Work out the finished part from the listing and answer in its coordinate system (mm). Coordinates: 2 decimals unless noted, no trailing zeros. Order: outer loops, then holes, each group sorted by start corner. A loop starts at its lowest first (then second) coordinate and runs counter-clockwise, first axis right, second up. Notation, with made-up numbers: (62.5, 55.5) - (102.5, 55.5) arc R18 ccw to (102.5, 59.5) - close; hole circle Ø5 at (88.25, 83). An arc over 180 degrees is marked (long way). Answer as a JSON object with one key per item and string values. Group by question number.
1) Section A-A (y = -0.95) is taken. Give the vertices of the cut face in (x, z) (1 decimal).
2) Find the intervals of material crossed by line 1 along X through (y, z) = (-0.1, 0); line 2 along X through (y, z) = (0.5, 0.75); line 3 along Z through (x, y) = (3.5, 0.9), in increasing order.
3) The mould has two halves that part along X. Classify faces 1 (the face through (-0.966, 0.015, -1.26)), 2 (the face through (3.563, -1.363, 2.046)), 3 (the face through (-3.962, 0, 0)), 4 (the face through (0.01, 1.363, 4.109)): released by +X, released by -X, zero draft, split by the parting line, or undercut.
4) This flat-tipped pin is pushed along its axis until it touches: P1, Ø3, axis at x = 0, z = 0, coming from the +Y side. Where does it stop, or does it pass through?
from build123d import *

# Parameters (mm, degrees)
BOSS_EXTRUDE1_DEPTH = 1.4478
SKETCH2_R           = 1.5875
CUT_EXTRUDE1_DEPTH  = 7.709639692
CHAMFER2_SIZE       = 0.381


with BuildPart() as part:
    # Sketch1 → Boss-Extrude1 (new, symmetric)
    with BuildSketch(Plane(origin=(0, 0, 0), x_dir=(1, 0, 0), z_dir=(0, 1, 0))):
        Polygon((0, -4.575385413), (3.9624, -2.287692707), (3.9624, 2.287692707), (0, 4.575385413), (-3.9624, 2.287692707), (-3.9624, -2.287692707), align=None)
    extrude(amount=BOSS_EXTRUDE1_DEPTH, both=True)

    # Sketch2 → Cut-Extrude1 (cut, through all)
    with BuildSketch(Plane(origin=(0, 1.4478, 0), x_dir=(1, 0, 0), z_dir=(0, 1, 0))):
        with Locations(Location((0, 0, 0), (0, 0, 270))):
            Circle(SKETCH2_R)
    extrude(amount=-CUT_EXTRUDE1_DEPTH, mode=Mode.SUBTRACT)

    # Sketch3 → Cut-Revolve2 (revolve, cut)
    with BuildSketch(Plane(origin=(0, 0, 0), x_dir=(0, 0, -1), z_dir=(1, 0, 0))):
        Polygon((-4.575385413, -1.4478), (-4.575385413, -1.093892707), (-3.9624, -1.4478), align=None)
    cut_revolve2 = revolve(axis=Axis((0, 0, 0), (0, -1, 0)), mode=Mode.SUBTRACT)

    # Mirror2: Cut-Revolve2 across plane
    add(cut_revolve2.mirror(Plane.ZX), mode=Mode.SUBTRACT)

    # Chamfer2
    chamfer2_edges = [part.edges().sort_by_distance(p)[0] for p in [
        (0, -1.4478, -1.5875),
        (0, 1.4478, -1.5875),
    ]]
    chamfer(chamfer2_edges, length=CHAMFER2_SIZE)


solid = part.part
Report:
{
 "1": {"outline": "(-4, -2.3) - (0, -4.6) - (4, -2.3) - (4, 2.3) - (0, 4.6) - (-4, 2.3) - close; hole circle Ø3.2 at (0, 0)"},
 "2": {"line 1": "x = -3.96 to -1.59, 1.59 to 3.96", "line 2": "x = -3.96 to -1.4, 1.4 to 3.96", "line 3": "z = -2.55 to 2.55"},
 "3": {"face 1": "undercut", "face 2": "released by +X", "face 3": "released by -X", "face 4": "split by the parting line"},
 "4": {"P1": "passes through"}
}
